The listing builds one solid part. Answer for the finished solid, in the listing's coordinates (mm). A direction names the side the tool comes from. Give positions to 0.01 mm unless a question says otherwise; leave off trailing zeros. Order: outer loops, then holes, each group sorted by start corner. A loop starts at its lowest first (then second) coordinate and runs counter-clockwise, first axis right, second up. Notation, with made-up numbers: (-23.75, 50) - (28.25, 50) arc R32 cw to (28.25, 81) - close; hole circle Ø2 at (-27.75, -24). An arc over 180 degrees is marked (long way). Answer in a Markdown table with one row per item.
from build123d import *

# Parameters (mm, degrees)
BOSS_EXTRU_1_DEPTH = 67.2
BOSS_EXTRU_2_DEPTH = 1.6
ESQUISSE3_R        = 1.8
BOSS_EXTRU_3_DEPTH = 10


with BuildPart() as part:
    # Esquisse1 → Boss.-Extru.1 (new, symmetric)
    with BuildSketch(Plane(origin=(0, 0, 0), x_dir=(1, 0, 0), z_dir=(0, 1, 0))):
        with BuildLine():
            Line((-11.55, 12.3), (11.55, 12.3))
            ThreePointArc((11.55, 12.3), (23.85, 0), (11.55, -12.3))
            Line((11.55, -12.3), (-11.55, -12.3))
            ThreePointArc((-11.55, -12.3), (-23.85, 0), (-11.55, 12.3))
        make_face()
    extrude(amount=BOSS_EXTRU_1_DEPTH, both=True)

    # Esquisse2 → Boss.-Extru.2 (add)
    with BuildSketch(Plane(origin=(0, 67.2, 0), x_dir=(1, 0, 0), z_dir=(0, 1, 0))):
        with BuildLine():
            Line((-10.9, 6.1), (10.9, 6.1))
            ThreePointArc((10.9, 6.1), (17, 0), (10.9, -6.1))
            Line((10.9, -6.1), (-10.9, -6.1))
            ThreePointArc((-10.9, -6.1), (-17, 0), (-10.9, 6.1))
        make_face()
    extrude(amount=BOSS_EXTRU_2_DEPTH)

    # Esquisse3 → Boss.-Extru.3 (add)
    with BuildSketch(Plane(origin=(0, 68.8, 0), x_dir=(1, 0, 0), z_dir=(0, 1, 0))):
        with Locations(Location((-1.85, 0, 0), (0, 0, 270))):
            Circle(ESQUISSE3_R)
        with Locations(Location((1.85, 0, 0), (0, 0, 90))):
            Circle(ESQUISSE3_R)
    extrude(amount=BOSS_EXTRU_3_DEPTH)


solid = part.part
Item 1: Find section C-C on x = -1.85. Write down the section's boundary in (y, z).
Answer block:
| item | result |
|---|---|
| outline | (-67.2, -12.3) - (67.2, -12.3) - (67.2, -6.1) - (68.8, -6.1) - (68.8, -1.8) - (78.8, -1.8) - (78.8, 1.8) - (68.8, 1.8) - (68.8, 6.1) - (67.2, 6.1) - (67.2, 12.3) - (-67.2, 12.3) - close |
Item 2: Find section A-A on z = 0. Write down the section's boundary in (x, y), then the cut area to 3 significant figures.
Answer block:
| item | result |
|---|---|
| outline | (-23.85, -67.2) - (23.85, -67.2) - (23.85, 67.2) - (17, 67.2) - (17, 68.8) - (3.65, 68.8) - (3.65, 78.8) - (0.05, 78.8) - (0.05, 68.8) - (-0.05, 68.8) - (-0.05, 78.8) - (-3.65, 78.8) - (-3.65, 68.8) - (-17, 68.8) - (-17, 67.2) - (-23.85, 67.2) - close |
| area | 6,540 mm² |
Item 3: Find section B-B on x = 5.5. Write down the section's boundary in (y, z), then the cut area to 3 significant figures.
Answer block:
| item | result |
|---|---|
| outline | (-67.2, -12.3) - (67.2, -12.3) - (67.2, -6.1) - (68.8, -6.1) - (68.8, 6.1) - (67.2, 6.1) - (67.2, 12.3) - (-67.2, 12.3) - close |
| area | 3,330 mm² |
Item 4: Which of the six approach directions +Z, -Z, +X, -X, +Y, -Y give full straight-line access (tool end or side, diameter ignored) to faces 4 (the face through (-17, 68, 0)), 5 (the face through (17, 68, 0)), 6 (the face through (0, 67.2, 8))?
Answer block:
| item | result |
|---|---|
| face 4 | -X, +Y |
| face 5 | +X, +Y |
| face 6 | +Y |
Item 5: Consider line 1 (Y direction, x = 16, z = 9.5); line 2 (Y direction, x = 6, z = -5.25); line 3 (X direction, y = 33, z = 6.25). Determine where each line is inside the solid, lowest interval first.
Answer block:
| item | result |
|---|---|
| line 1 | -67.2 to 67.2 |
| line 2 | -67.2 to 68.8 |
| line 3 | -22.14 to 22.14 |
Item 6: Each of these flat-tipped pins is pushed along its axis until it touches: P1, Ø3.5, axis at x = -4.5, z = 0, coming from the +Y side; P2, Ø0.8, axis at x = -2, y = 68, coming from the +Z side; P3, Ø1, axis at x = 15.5, y = -24, coming from the -Z side; P4, Ø1, axis at y = 25.5, z = -7, coming from the -X side. Where does it stop, or does it pass through?
Answer block:
| item | result |
|---|---|
| P1 | y = 78.8 |
| P2 | z = 6.1 |
| P3 | z = -11.81 |
| P4 | x = -21.99 |
Item 7: Find section D-D on y = -22. Write down the section's boundary in (x, z).
Answer block:
| item | result |
|---|---|
| outline | (-11.55, -12.3) - (11.55, -12.3) arc R12.3 ccw to (11.55, 12.3) - (-11.55, 12.3) arc R12.3 ccw to start |
Item 8: Determine the mould class of faces 1 (the face through (2, 78.8, 0)), 2 (the face through (-23.847, 0.941, 0.27)), 3 (the face through (2.539, 73.73, -1.663)) for opening direction X: pulls with the +X half, pulls with the -X half, needs draft (parallel to the pull), parting line crosses it, or undercut.
Answer block:
| item | result |
|---|---|
| face 1 | needs draft |
| face 2 | pulls with the -X half |
| face 3 | undercut |
